The listing builds one solid part. Answer for the finished solid, in the listing's coordinates (mm). Face numbers are marked on the shaded views. A direction names the side the tool comes from. Round coordinates to 2 decimals unless told otherwise and drop trailing zeros. Write each loop counter-clockwise with the first axis right and the second up, starting at its lowest first coordinate (ties: lowest second). Pieces come first, ordered by that corner, then holes. Notation, with made-up numbers: (76.5, 32.25) - (124.5, 32.25) arc R23 ccw to (124.5, 61.25) - close; hole circle Ø11 at (-32, 2). An arc over 180 degrees is marked (long way). Answer as CSV lines item,"result". Start each with the question number.
Item 1: A cutting plane is placed at C-C on z = 1.3. State how many separate pieces and enclosed holes the cut face has, and give its area (3 significant figures).
Item 2: A cutting plane is placed at A-A on x = -33. Determine the outline of the cut face in (y, z).
Item 3: Flat-ended cylindrical pins translate along their axes: pin 1 (1.5 mm diameter, centred on x = 4, z = 3, fed in from -Y); pin 2 (0.5 mm diameter, centred on y = 0.5, z = 1.5, fed in from +X). Find the tip coordinate at first contact, or state that the pin passes through.
Item 4: A cutting plane is placed at B-B on y = -31. Determine the outline of the cut face in (x, z), and give its area (3 significant figures).
Item 5: Straight lines are drawn through the part: line 1 along X through (y, z) = (-1.5, 3.55); line 2 along X through (y, z) = (1.5, 4.3); line 3 along Y through (x, z) = (0, 1.35). For each, find the intervals that lie inside material, in ascending order. Write a range as [from, to].
Item 6: For a pull along Z with two mould halves and no side action, classify the marked faces 4, 5 and 6 as pulls with the +Z half, pulls with the -Z half, needs draft (parallel to the pull), parting line crosses it, or undercut.
Item 7: Which of the six approach directions +Z, -Z, +X, -X, +Y, -Y give full straight-line access (tool end or side, diameter ignored) to the marked faces 1, 2 and 3?
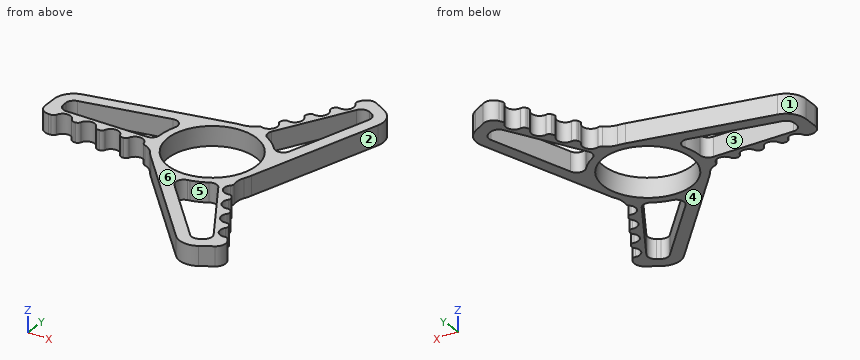
```python
from build123d import *

# Parameters (mm, degrees)
F0_R     = 11
F1_DEPTH = 4.83


with BuildPart() as f1:
    # F0 (on Top) → F1 (new body)
    with BuildSketch(Plane.XY):
        with BuildLine():
            ThreePointArc((-36.01296, 5.824847), (-38.877164, 4.085682), (-40, 0.928531))
            Line((-40, 0.928531), (-40, -2.5))
            ThreePointArc((-40, -2.5), (-39.267767, -4.267767), (-37.5, -5))
            Line((-37.5, -5), (-36.828427, -5))
            ThreePointArc((-36.828427, -5), (-36.251077, -4.816497), (-35.885618, -4.333333))
            ThreePointArc((-35.885618, -4.333333), (-34, -3), (-32.114382, -4.333333))
            ThreePointArc((-32.114382, -4.333333), (-31.748923, -4.816497), (-31.171573, -5))
            Line((-31.171573, -5), (-30.828573, -5))
            ThreePointArc((-30.828573, -5), (-30.251193, -4.816476), (-29.88574, -4.333265))
            ThreePointArc((-29.88574, -4.333265), (-28.000073, -2.999794), (-26.114406, -4.333265))
            ThreePointArc((-26.114406, -4.333265), (-25.748953, -4.816476), (-25.171573, -5))
            Line((-25.171573, -5), (-24.828427, -5))
            ThreePointArc((-24.828427, -5), (-24.251077, -4.816497), (-23.885618, -4.333333))
            ThreePointArc((-23.885618, -4.333333), (-22, -3), (-20.114382, -4.333333))
            ThreePointArc((-20.114382, -4.333333), (-19.748923, -4.816497), (-19.171573, -5))
            Line((-19.171573, -5), (-18.828427, -5))
            ThreePointArc((-18.828427, -5), (-18.251077, -4.816497), (-17.885618, -4.333333))
            ThreePointArc((-17.885618, -4.333333), (-15.89445, -3.002787), (-14.054617, -4.535797))
            ThreePointArc((-14.054617, -4.535797), (-13.818534, -4.980014), (-13.396043, -5.253079))
            ThreePointArc((-13.396043, -5.253079), (-11.938126, -6.021537), (-10.809232, -7.222222))
            ThreePointArc((-10.809232, -7.222222), (-10.283299, -7.953223), (-9.70802, -8.64606))
            Line((-9.70802, -8.64606), (12.962014, -34.100562))
            ThreePointArc((12.962014, -34.100562), (15.900278, -35.711453), (19.195868, -35.105282))
            Line((19.195868, -35.105282), (22.165064, -33.391016))
            ThreePointArc((22.165064, -33.391016), (23.329878, -31.873), (23.080127, -29.975953))
            Line((23.080127, -29.975953), (22.744341, -29.394353))
            ThreePointArc((22.744341, -29.394353), (22.296747, -28.986105), (21.695586, -28.91119))
            ThreePointArc((21.695586, -28.91119), (19.598076, -27.944864), (19.809968, -25.645204))
            ThreePointArc((19.809968, -25.645204), (20.04567, -25.087126), (19.915913, -24.495374))
            Line((19.915913, -24.495374), (19.744413, -24.198327))
            ThreePointArc((19.744413, -24.198327), (19.296787, -23.790064), (18.695587, -23.715177))
            ThreePointArc((18.695587, -23.715177), (16.597934, -22.748877), (16.80992, -20.449107))
            ThreePointArc((16.80992, -20.449107), (17.045667, -19.89101), (16.915913, -19.299222))
            Line((16.915913, -19.299222), (16.744341, -19.002049))
            ThreePointArc((16.744341, -19.002049), (16.296747, -18.5938), (15.695586, -18.518885))
            ThreePointArc((15.695586, -18.518885), (13.598076, -17.552559), (13.809968, -15.252899))
            ThreePointArc((13.809968, -15.252899), (14.04567, -14.694821), (13.915913, -14.103069))
            Line((13.915913, -14.103069), (13.744341, -13.805896))
            ThreePointArc((13.744341, -13.805896), (13.296747, -13.397648), (12.695586, -13.322733))
            ThreePointArc((12.695586, -13.322733), (10.547715, -12.263604), (10.955424, -9.903757))
            ThreePointArc((10.955424, -9.903757), (11.222086, -9.477195), (11.247321, -8.974774))
            ThreePointArc((11.247321, -8.974774), (11.183867, -7.327952), (11.659244, -5.749959))
            ThreePointArc((11.659244, -5.749959), (12.029343, -4.928987), (12.341717, -4.084362))
            Line((12.341717, -4.084362), (23.050946, 28.275715))
            ThreePointArc((23.050946, 28.275715), (22.976886, 31.625771), (20.804132, 34.17675))
            Line((20.804132, 34.17675), (17.834936, 35.891016))
            ThreePointArc((17.834936, 35.891016), (15.937889, 36.140767), (14.419873, 34.975953))
            Line((14.419873, 34.975953), (14.084087, 34.394353))
            ThreePointArc((14.084087, 34.394353), (13.95433, 33.802602), (14.190032, 33.244524))
            ThreePointArc((14.190032, 33.244524), (14.401924, 30.944864), (12.304414, 29.978537))
            ThreePointArc((12.304414, 29.978537), (11.703253, 29.903622), (11.255659, 29.495374))
            Line((11.255659, 29.495374), (11.084159, 29.198327))
            ThreePointArc((11.084159, 29.198327), (10.954406, 28.606539), (11.190153, 28.048442))
            ThreePointArc((11.190153, 28.048442), (11.402139, 25.748671), (9.304486, 24.782371))
            ThreePointArc((9.304486, 24.782371), (8.703286, 24.707485), (8.255659, 24.299222))
            Line((8.255659, 24.299222), (8.084087, 24.002049))
            ThreePointArc((8.084087, 24.002049), (7.95433, 23.410297), (8.190032, 22.852219))
            ThreePointArc((8.190032, 22.852219), (8.401924, 20.552559), (6.304414, 19.586232))
            ThreePointArc((6.304414, 19.586232), (5.703253, 19.511317), (5.255659, 19.103069))
            Line((5.255659, 19.103069), (5.084087, 18.805896))
            ThreePointArc((5.084087, 18.805896), (4.95433, 18.214144), (5.190032, 17.656066))
            ThreePointArc((5.190032, 17.656066), (5.346735, 15.266391), (3.099193, 14.439554))
            ThreePointArc((3.099193, 14.439554), (2.596449, 14.457209), (2.148721, 14.227853))
            ThreePointArc((2.148721, 14.227853), (0.754259, 13.349489), (-0.850012, 12.972181))
            ThreePointArc((-0.850012, 12.972181), (-1.746044, 12.88221), (-2.633697, 12.730422))
            Line((-2.633697, 12.730422), (-36.01296, 5.824847))
        make_face()
        with BuildLine():
            ThreePointArc((6.5, -11.25833), (8.017638, -11.058529), (9.232051, -11.990381))
            Line((9.232051, -11.990381), (19.232051, -29.310889))
            ThreePointArc((19.232051, -29.310889), (19.431852, -30.828527), (18.5, -32.04294))
            Line((18.5, -32.04294), (17.695868, -32.507206))
            ThreePointArc((17.695868, -32.507206), (16.377632, -32.749674), (15.202327, -32.105318))
            Line((15.202327, -32.105318), (0.971231, -16.126274))
            ThreePointArc((0.971231, -16.126274), (0.578639, -14.130903), (2.136136, -12.823296))
            ThreePointArc((2.136136, -12.823296), (2.385369, -12.779281), (2.633697, -12.730422))
            ThreePointArc((2.633697, -12.730422), (4.625783, -12.149162), (6.5, -11.25833))
        make_face(mode=Mode.SUBTRACT)
        Circle(F0_R, mode=Mode.SUBTRACT)
        with BuildLine():
            ThreePointArc((-14.451378, 7.222027), (-12.527041, 6.564336), (-12.173368, 4.5617))
            ThreePointArc((-12.173368, 4.5617), (-12.791673, 2.317996), (-13, 0))
            ThreePointArc((-13, 0), (-13.585786, -1.414214), (-15, -2))
            Line((-15, -2), (-35, -2))
            ThreePointArc((-35, -2), (-36.414214, -1.414214), (-37, 0))
            Line((-37, 0), (-37, 0.928531))
            ThreePointArc((-37, 0.928531), (-36.550866, 2.191391), (-35.405184, 2.887058))
            Line((-35.405184, 2.887058), (-14.451378, 7.222027))
        make_face(mode=Mode.SUBTRACT)
        with BuildLine():
            ThreePointArc((6.5, 11.25833), (5.568148, 12.472743), (5.767949, 13.990381))
            Line((5.767949, 13.990381), (15.767949, 31.310889))
            ThreePointArc((15.767949, 31.310889), (16.982362, 32.242741), (18.5, 32.04294))
            Line((18.5, 32.04294), (19.304132, 31.578674))
            ThreePointArc((19.304132, 31.578674), (20.173234, 30.558282), (20.202857, 29.21826))
            Line((20.202857, 29.21826), (13.480148, 8.904247))
            ThreePointArc((13.480148, 8.904247), (11.948402, 7.566568), (10.037232, 8.261596))
            ThreePointArc((10.037232, 8.261596), (8.40328, 9.918915), (6.5, 11.25833))
        make_face(mode=Mode.SUBTRACT)
    extrude(amount=F1_DEPTH)


solid = f1.part
```
Geometry says:
1,separate pieces,"1"
1,enclosed holes,"4"
1,area,"662 mm^2"
2,outline,"(-3.27, 0) - (-2, 0) - (-2, 4.83) - (-3.27, 4.83) - close; (3.38, 0) - (6.45, 0) - (6.45, 4.83) - (3.38, 4.83) - close"
3,pin 1,"stops at y = -24.88"
3,pin 2,"stops at x = 13.94"
4,outline,"(10.2, 0) - (14.22, 0) - (14.22, 4.83) - (10.2, 4.83) - close; (19.38, 0) - (23.4, 0) - (23.4, 4.83) - (19.38, 4.83) - close"
4,area,"38.9 mm^2"
5,line 1,"x = [-40, -36.32], [-13.68, -10.9], [10.9, 13.2]"
5,line 2,"x = [-39.97, -36.92], [-12.91, -10.9], [10.9, 14.19]"
5,line 3,"y = [-19.55, -11], [11, 13.1]"
6,face 4,"pulls with the -Z half"
6,face 5,"needs draft"
6,face 6,"pulls with the +Z half"
7,face 1,"+Z, -Z, -X, +Y"
7,face 2,"+Z, -Z, +X"
7,face 3,"+Z, -Z"
